from build123d import *

# Parameters (mm, degrees)
BOSS_EXTRUDE1_DEPTH     = 12.7
CUT_EXTRUDE2_DEPTH      = 33.274
CUT_EXTRUDE2_DEPTH_BACK = 25.4
CUT_EXTRUDE3_DEPTH      = 6.35
CUT_EXTRUDE4_DEPTH      = 6.35
CUT_EXTRUDE5_DEPTH      = 6.35


with BuildPart() as part:
    # Sketch1 → Boss-Extrude1 (new body)
    with BuildSketch(Plane(origin=(0, 0, 0), x_dir=(1, 0, 0), z_dir=(0, 1, 0))):
        Polygon((-69.85, 0), (0, 0), (69.85, 0), (69.85, 38.1), (50.8, 38.1), (31.75, 139.7), (44.45, 139.7), (44.45, 158.75), (0, 158.75), (-44.45, 158.75), (-44.45, 139.7), (-31.75, 139.7), (-50.8, 38.1), (-69.85, 38.1), align=None)
    extrude(amount=BOSS_EXTRUDE1_DEPTH)

    # Sketch3 → Cut-Extrude2 (cut, two sides)
    with BuildSketch(Plane(origin=(0, 0, 0), x_dir=(1, 0, 0), z_dir=(0, 1, 0))) as cut_extrude2_sk:
        Polygon((0, 38.209887603), (-38.1, 38.209887603), (-19.05, 139.809887603), (0, 139.809887603), (19.05, 139.809887603), (38.1, 38.209887603), align=None)
    extrude(amount=CUT_EXTRUDE2_DEPTH, mode=Mode.SUBTRACT)
    extrude(cut_extrude2_sk.sketch, amount=-CUT_EXTRUDE2_DEPTH_BACK, mode=Mode.SUBTRACT)

    # Sketch4 → Cut-Extrude3 (cut)
    with BuildSketch(Plane(origin=(0, 12.7, 0), x_dir=(1, 0, 0), z_dir=(0, 1, 0))):
        Polygon((-38.1, 30.497184411), (-26.396078431, 30.497184411), (-26.396078431, 24.528945876), (-34.833932912, 24.528945876), (-34.833932912, 5.183620969), (-38.1, 5.183620969), (-41.366067088, 5.183620969), (-41.366067088, 24.528945876), (-49.803921569, 24.528945876), (-49.803921569, 30.497184411), align=None)
    extrude(amount=-CUT_EXTRUDE3_DEPTH, mode=Mode.SUBTRACT)

    # Sketch5 → Cut-Extrude4 (cut)
    with BuildSketch(Plane(origin=(0, 12.7, 0), x_dir=(1, 0, 0), z_dir=(0, 1, 0))):
        with BuildLine():
            Line((-9.055258467, 5.595223627), (-9.055258467, 30.908787069))
            Line((-9.055258467, 30.908787069), (-0.411602658, 30.908787069))
            ThreePointArc((-0.411602658, 30.908787069), (5.762437206, 24.734747205), (-0.411602658, 18.560707341))
            ThreePointArc((-0.411602658, 18.560707341), (6.071139199, 12.077965484), (-0.411602658, 5.595223627))
            Line((-0.411602658, 5.595223627), (-9.055258467, 5.595223627))
        make_face()
        with BuildLine():
            Line((-3.704423918, 9.917051531), (-3.704423918, 15.885290066))
            ThreePointArc((-3.704423918, 15.885290066), (-0.720304651, 12.901170799), (-3.704423918, 9.917051531))
        make_face(mode=Mode.SUBTRACT)
        with BuildLine():
            Line((-3.704423918, 22.05932993), (-3.704423918, 27.821767137))
            ThreePointArc((-3.704423918, 27.821767137), (-0.823205315, 24.940548533), (-3.704423918, 22.05932993))
        make_face(mode=Mode.SUBTRACT)
    extrude(amount=-CUT_EXTRUDE4_DEPTH, mode=Mode.SUBTRACT)

    # Sketch6 → Cut-Extrude5 (cut)
    with BuildSketch(Plane(origin=(0, 12.7, 0), x_dir=(1, 0, 0), z_dir=(0, 1, 0))):
        Polygon((26.548371415, 5.595223627), (33.751417923, 5.595223627), (33.751417923, 23.769556722), (41.160265759, 23.769556722), (41.160265759, 5.595223627), (48.363312267, 5.595223627), (48.363312267, 30.908787069), (26.548371415, 30.908787069), align=None)
    extrude(amount=-CUT_EXTRUDE5_DEPTH, mode=Mode.SUBTRACT)


solid = part.part
The model under review builds one solid part; all positions refer to its coordinate system, in mm. A direction names the side the tool comes from. Round coordinates to 2 decimals unless told otherwise and drop trailing zeros. Loops run counter-clockwise (first coordinate to the right, second up) from the corner with the lowest first, then second, coordinate; pieces in that order, holes last. Notation, with made-up numbers: (22.25, -14) -> (45.25, -14) arc R15 cw to (45.25, -2) -> close; hole circle Ø5 at (24, 85). An arc over 180 degrees is marked (long way). One line per question, with ' | ' between items. Start each with the question number.
Item 1: Draft analysis for pull direction X (two halves, no side actions). For faces 1 (the face through (1, 6, -158.75)), 2 (the face through (-1, 6.35, -18)), 3 (the face through (44.45, 6, -149)), 4 (the face through (-69.85, 6, -19)), state which applies: +X half, -X half, draft (parallel to the pull), parting line (faces both ways), or undercut.
Item 2: Machinability: for faces 5 (the face through (41.41, 6.26, -88.19)), 6 (the face through (37, 10, -23.77)), 7 (the face through (28.44, 6.26, -89.72)), which of the approach directions +Z, -Z, +X, -X, +Y, -Y give a long, thin tool a straight path to every point of the face, cutting with its end or side? Answer none if there is none.
Item 3: Add section A-A, the plane x = -14.5. Write out the cut boundary in (y, z), then the cut area to 3 significant figures.
Item 4: Add section B-B, the plane y = 3.25. Write out the cut boundary in (x, z).
Item 5: Wall thickness on line 1 along Z through (x, y) = (-1.5, 3.5); line 2 along Z through (x, y) = (-5, 8.5); line 3 along Z through (x, y) = (-57, 10.5): over which ranges is each line inside the solid? List them lowest first. Write a range as [from, to].
Item 6: For pin 1 (4 mm diameter, centred on y = 8, z = -152.5, fed in from -X), flat-tipped, find the tip position at first contact; note if it passes through.
Item 7: Add section C-C, the plane z = -120. Write out the cut boundary in (x, y).
Item 8: Add section D-D, the plane z = -145. Write out the cut boundary in (x, y).
Return value:
1) face 1: draft | face 2: undercut | face 3: +X half | face 4: -X half
2) face 5: +X, +Y, -Y | face 6: +Y | face 7: +Y, -Y
3) outline: (0, -158.75) -> (12.7, -158.75) -> (12.7, -139.81) -> (0, -139.81) -> close; (0, -38.21) -> (12.7, -38.21) -> (12.7, 0) -> (0, 0) -> close | area: 726 mm2
4) outline: (-69.85, -38.1) -> (-50.8, -38.1) -> (-31.75, -139.7) -> (-44.45, -139.7) -> (-44.45, -158.75) -> (44.45, -158.75) -> (44.45, -139.7) -> (31.75, -139.7) -> (50.8, -38.1) -> (69.85, -38.1) -> (69.85, 0) -> (-69.85, 0) -> close; hole (-38.1, -38.21) -> (-19.05, -139.81) -> (19.05, -139.81) -> (38.1, -38.21) -> close
5) line 1: z = [-158.75, -139.81], [-38.21, 0] | line 2: z = [-158.75, -139.81], [-38.21, -30.91], [-5.6, 0] | line 3: z = [-38.1, 0]
6) pin 1: stops at x = -44.45
7) outline: (-35.44, 0) -> (-22.76, 0) -> (-22.76, 12.7) -> (-35.44, 12.7) -> close; (22.76, 0) -> (35.44, 0) -> (35.44, 12.7) -> (22.76, 12.7) -> close
8) outline: (-44.45, 0) -> (44.45, 0) -> (44.45, 12.7) -> (-44.45, 12.7) -> close
